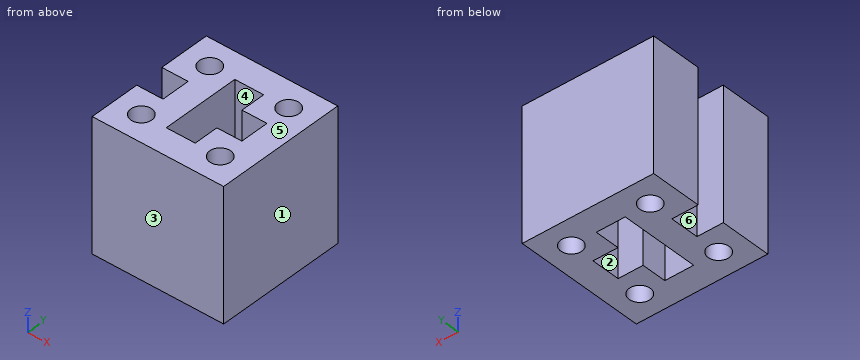
from build123d import *

# Parameters (mm, degrees)
F0_R     = 20
F1_DEPTH = 125


with BuildPart() as f1:
    # F0 (on Top) → F1 (new body, symmetric)
    with BuildSketch(Plane.XY):
        Polygon((125, -125), (125, 125), (-125, 125), (-125, 27.5), (-75, 27.5), (-75, -27.5), (-125, -27.5), (-125, -125), align=None)
        with Locations((-75, -75)):
            Circle(F0_R, mode=Mode.SUBTRACT)
        with Locations((75, -75)):
            Circle(F0_R, mode=Mode.SUBTRACT)
        with Locations((-75, 75)):
            Circle(F0_R, mode=Mode.SUBTRACT)
        Polygon((-27.5, -75), (-27.5, 75), (27.5, 75), (27.5, 27.5), (75, 27.5), (75, -27.5), (27.5, -27.5), (27.5, -75), align=None, mode=Mode.SUBTRACT)
        with Locations((75, 75)):
            Circle(F0_R, mode=Mode.SUBTRACT)
    extrude(amount=F1_DEPTH, both=True)


solid = f1.part
Design review of the part built by this model. Coordinates are the model's own, in mm. Face numbers are marked on the shaded views. A direction names the side the tool comes from. Round coordinates to 2 decimals unless told otherwise and drop trailing zeros. Loops run counter-clockwise (first coordinate to the right, second up) from the corner with the lowest first, then second, coordinate; pieces in that order, holes last. Notation, with made-up numbers: (11, 9) -> (61, 9) arc R11 ccw to (61, 13) -> close; hole circle Ø4 at (-18, -32). An arc over 180 degrees is marked (long way). Use one line per item in the form item = value. Start each with the question number.
Q1. We need section B-B on z = 70. Give the boundary of the cut face in (x, y), then the cut area to 3 significant figures.
Q2. For pin 1 Ø16.5 at (y, z) = (4, 7.5) entering from -X; pin 2 Ø10 at (x, y) = (-82, -12) entering from -Z, all flat-tipped, find the tip position at first contact; note any pin that passes through.
Q3. Machinability: for the marked faces 4, 5 and 6, which of the approach directions +Z, -Z, +X, -X, +Y, -Y give a long, thin tool a straight path to every point of the face, cutting with its end or side? Answer none if there is none.
Q4. Wall thickness on line 1 along Y through (x, z) = (5.5, -76); line 2 along X through (y, z) = (-78, 18); line 3 along Y through (x, z) = (-67.5, -88): over which ranges is each line inside the solid? List them lowest first. Write a range as [from, to].
Q5. We need section A-A on y = 36.5. Give the boundary of the cut face in (x, z), then the cut area to 4 significant figures.
Q6. We need section C-C on y = -67. Give the boundary of the cut face in (x, z).
Q7. Draft analysis for pull direction Y (two halves, no side actions). For the marked faces 1, 2 and 3, state which applies: +Y half, -Y half, draft (parallel to the pull), parting line (faces both ways), or undercut.
Q8. We need section D-D on y = 61.5. Give the boundary of the cut face in (x, z), then the cut area to 3 significant figures.
Calculated:
q1.outline = (-125, -125) -> (125, -125) -> (125, 125) -> (-125, 125) -> (-125, 27.5) -> (-75, 27.5) -> (-75, -27.5) -> (-125, -27.5) -> close; hole circle Ø40 at (-75, -75); hole circle Ø40 at (-75, 75); hole (-27.5, -75) -> (27.5, -75) -> (27.5, -27.5) -> (75, -27.5) -> (75, 27.5) -> (27.5, 27.5) -> (27.5, 75) -> (-27.5, 75) -> close; hole circle Ø40 at (75, -75); hole circle Ø40 at (75, 75)
q1.area = 43,900 mm²
q2.pin_1 = -75
q2.pin_2 = through
q3.face_4 = +Z, -Z
q3.face_5 = +Z, +X, -X, +Y, -Y
q3.face_6 = +Z, -Z, -X
q4.line_1 = [-125, -75], [75, 125]
q4.line_2 = [-125, -94.77], [-55.23, 55.23], [94.77, 125]
q4.line_3 = [-125, -93.54], [-56.46, 56.46], [93.54, 125]
q5.outline = (-125, -125) -> (-27.5, -125) -> (-27.5, 125) -> (-125, 125) -> close; (27.5, -125) -> (125, -125) -> (125, 125) -> (27.5, 125) -> close
q5.area = 48,750 mm²
q6.outline = (-125, -125) -> (-93.33, -125) -> (-93.33, 125) -> (-125, 125) -> close; (-56.67, -125) -> (-27.5, -125) -> (-27.5, 125) -> (-56.67, 125) -> close; (27.5, -125) -> (56.67, -125) -> (56.67, 125) -> (27.5, 125) -> close; (93.33, -125) -> (125, -125) -> (125, 125) -> (93.33, 125) -> close
q7.face_1 = draft
q7.face_2 = undercut
q7.face_3 = -Y half
q8.outline = (-125, -125) -> (-89.76, -125) -> (-89.76, 125) -> (-125, 125) -> close; (-60.24, -125) -> (-27.5, -125) -> (-27.5, 125) -> (-60.24, 125) -> close; (27.5, -125) -> (60.24, -125) -> (60.24, 125) -> (27.5, 125) -> close; (89.76, -125) -> (125, -125) -> (125, 125) -> (89.76, 125) -> close
q8.area = 34,000 mm²
